```python
from build123d import *

# Parameters (mm, degrees)
BOSS_EXTRUDE1_DEPTH = 10
SKETCH2_R           = 5
BOSS_EXTRUDE2_DEPTH = 10


with BuildPart() as part:
    # Sketch1 → Boss-Extrude1 (new body)
    with BuildSketch(Plane(origin=(0, 0, 0), x_dir=(1, 0, 0), z_dir=(0, 1, 0))):
        with BuildLine():
            Line((8, 20), (8, -20))
            ThreePointArc((8, -20), (0, -28), (-8, -20))
            Line((-8, -20), (-8, 20))
            ThreePointArc((-8, 20), (0, 28), (8, 20))
        make_face()
    extrude(amount=BOSS_EXTRUDE1_DEPTH)

    # Sketch2 → Boss-Extrude2 (add)
    with BuildSketch(Plane.XZ):
        with Locations(Location((0, 20, 0), (0, 0, 90))):
            Circle(SKETCH2_R)
    extrude(amount=BOSS_EXTRUDE2_DEPTH)


solid = part.part
```
Here's how the part is built. I have some questions about the finished solid (model axes, mm). A direction names the side the tool comes from. Give positions to 0.01 mm unless a question says otherwise; leave off trailing zeros. Order: outer loops, then holes, each group sorted by start corner. A loop starts at its lowest first (then second) coordinate and runs counter-clockwise, first axis right, second up. Notation, with made-up numbers: M 77,-26 L 96,-26 A11 cw 96,-7 Z; hole C 49,72.25 d1. An arc over 180 degrees is marked long. Use a Markdown table: item, result. Add a question column.
1. Suppose I cut it at B-B (y = 2). List the corners of the cut face in (x, z) for me.
2. I need wall thicknesses on probe 1 along Y at (x, z) = (1, 4.5); probe 2 along Z at (x, y) = (-4.75, 5.5); probe 3 along X at (y, z) = (2.75, 21). Which ranges of each line are inside material? Lowest first, please. Write a range as from..to.
3. For pin 1 Ø6 at (x, z) = (-2, -22.5) entering from -Y; pin 2 Ø3 at (y, z) = (-2.5, 20) entering from +X, each with a flat end and sliding along its axis, tell me the tip position at first contact or that it passes through.
4. Suppose I cut it at C-C (z = -4). List the corners of the cut face in (x, y) for me, and give its area (3 significant figures).
5. On a 3-axis mill with a long thin cutter (end or side, diameter ignored), from which of +Z, -Z, +X, -X, +Y, -Y can I reach the whole of each face in a straight line? I mean faces 1 (the cylindrical face through (0, -5, 15)), 2 (the flat face through (0, 10, 0)). Say none if no direction works.
6. Suppose I cut it at A-A (x = 0). List the corners of the cut face in (y, z) for me.
7. Suppose I cut it at D-D (x = 2.25). List the corners of the cut face in (y, z) for me, and give its area (3 significant figures).
Results list:
| question | item | result |
|---|---|---|
| 1 | outline | M -8,-20 A8 ccw 8,-20 L 8,20 A8 ccw -8,20 Z |
| 2 | probe 1 | y = 0..10 |
| 2 | probe 2 | z = -26.44..26.44 |
| 2 | probe 3 | x = -7.94..7.94 |
| 3 | pin 1 | stops at y = 0 |
| 3 | pin 2 | stops at x = 5 |
| 4 | outline | M -8,0 L 8,0 L 8,10 L -8,10 Z |
| 4 | area | 160 mm² |
| 5 | face 1 | -Y |
| 5 | face 2 | +Z, -Z, +X, -X, +Y |
| 6 | outline | M -10,15 L 0,15 L 0,-28 L 10,-28 L 10,28 L 0,28 L 0,25 L -10,25 Z |
| 7 | outline | M -10,15.53 L 0,15.53 L 0,-27.68 L 10,-27.68 L 10,27.68 L 0,27.68 L 0,24.47 L -10,24.47 Z |
| 7 | area | 643 mm² |
